from build123d import *

# Parameters (mm, degrees)
SKETCH1_W                                = 152.4
SKETCH1_H                                = 228.6
BOSS_EXTRUDE1_DEPTH                      = 5.588
SKETCH2_R                                = 2.25
SKETCH2_W                                = 22
SKETCH2_H                                = 42
CUT_EXTRUDE1_DEPTH                       = 138.48511099
SKETCH6_R                                = 2.65
CUT_EXTRUDE2_DEPTH                       = 430.910746044
CUT_EXTRUDE3_DEPTH                       = 138.48511099
MIRROR1_AT_THE_SECOND_PLANE_COPY_1_DEPTH = 138.48511099
SKETCH8_R                                = 2.65
CUT_EXTRUDE4_DEPTH                       = 430.910746044
CUT_EXTRUDE5_DEPTH                       = 138.48511099
MIRROR2_AT_THE_SECOND_PLANE_COPY_1_DEPTH = 138.48511099
SKETCH10_W                               = 228.6
SKETCH10_H                               = 5.588
BOSS_EXTRUDE2_DEPTH                      = 25.4
SKETCH11_W                               = 22
SKETCH11_H                               = 42
CUT_EXTRUDE6_DEPTH                       = 154.030309887
CUT_EXTRUDE7_DEPTH                       = 154.030309887
MIRROR5_AT_THE_SECOND_PLANE_COPY_1_DEPTH = 154.030309887


with BuildPart() as part:
    # Sketch1 → Boss-Extrude1 (new body)
    with BuildSketch(Plane(origin=(0, 0, 0), x_dir=(1, 0, 0), z_dir=(0, 1, 0))):
        Rectangle(SKETCH1_W, SKETCH1_H)
    extrude(amount=BOSS_EXTRUDE1_DEPTH)

    # Sketch2 → Cut-Extrude1 (cut, through all)
    with BuildSketch(Plane(origin=(0, 5.588, 0), x_dir=(1, 0, 0), z_dir=(0, 1, 0))):
        with Locations(Location((64.145199836, -6.727348554, 0), (0, 0, 270))):
            Circle(SKETCH2_R)
        with Locations((74.145199836, -6.727348554)):
            Circle(SKETCH2_R)
        with Locations(Location((64.145199836, -54.727348554, 0), (0, 0, 270))):
            Circle(SKETCH2_R)
        with Locations((74.145199836, -54.727348554)):
            Circle(SKETCH2_R)
        with Locations((-74.023936008, -54.727348554)):
            Circle(SKETCH2_R)
        with Locations(Location((-64.023936008, -54.727348554, 0), (0, 0, 90))):
            Circle(SKETCH2_R)
        with Locations((-74.023936008, -6.727348554)):
            Circle(SKETCH2_R)
        with Locations(Location((-64.023936008, -6.727348554, 0), (0, 0, 90))):
            Circle(SKETCH2_R)
        with Locations((69.145199836, -30.727348554)):
            Rectangle(SKETCH2_W, SKETCH2_H)
        with Locations((-69.023936008, -30.727348554)):
            Rectangle(SKETCH2_W, SKETCH2_H)
    extrude(amount=-CUT_EXTRUDE1_DEPTH, mode=Mode.SUBTRACT)

    # Sketch6 → Cut-Extrude2 (cut, through all)
    with BuildSketch(Plane(origin=(-338.200209725, 5.588, 0), x_dir=(1, 0, 0), z_dir=(0, 1, 0))):
        with Locations(Location((404.400209725, 104.3, 0), (0, 0, 270))):
            Circle(SKETCH6_R)
    extrude(amount=-CUT_EXTRUDE2_DEPTH, mode=Mode.SUBTRACT)

    # Sketch7 → Cut-Extrude3 (cut, through all)
    with BuildSketch(Plane(origin=(0, 5.588, 0), x_dir=(1, 0, 0), z_dir=(0, 1, 0))):
        with BuildLine():
            Line((68.85, 105.377738503), (68.85, 97.377738503))
            ThreePointArc((68.85, 97.377738503), (66.2, 94.727738503), (63.55, 97.377738503))
            Line((63.55, 97.377738503), (63.55, 105.377738503))
            ThreePointArc((63.55, 105.377738503), (66.2, 108.027738503), (68.85, 105.377738503))
        make_face()
    cut_extrude3 = extrude(amount=-CUT_EXTRUDE3_DEPTH, mode=Mode.SUBTRACT)

    # Mirror1: Cut-Extrude3 across plane
    add(cut_extrude3.mirror(Plane.XY), mode=Mode.SUBTRACT)

    # Mirror1 at the second plane: Cut-Extrude3 across plane
    add(cut_extrude3.mirror(Plane(origin=(0, 0, 0), x_dir=(0, 0, 1), z_dir=(1, 0, 0))), mode=Mode.SUBTRACT)

    # Mirror1 at the second plane copy 1 sketc → Mirror1 at the second plane copy 1 (cut, through all)
    with BuildSketch(Plane(origin=(0, 5.588, 0), x_dir=(-1, 0, 0), z_dir=(0, 1, 0))):
        with BuildLine():
            Line((68.85, 105.377738503), (68.85, 97.377738503))
            ThreePointArc((68.85, 97.377738503), (66.2, 94.727738503), (63.55, 97.377738503))
            Line((63.55, 97.377738503), (63.55, 105.377738503))
            ThreePointArc((63.55, 105.377738503), (66.2, 108.027738503), (68.85, 105.377738503))
        make_face()
    extrude(amount=-MIRROR1_AT_THE_SECOND_PLANE_COPY_1_DEPTH, mode=Mode.SUBTRACT)

    # Sketch8 → Cut-Extrude4 (cut, through all)
    with BuildSketch(Plane(origin=(-338.200209725, 5.588, 0), x_dir=(1, 0, 0), z_dir=(0, 1, 0))):
        with Locations(Location((381.82832329, 70.726177663, 0), (0, 0, 270))):
            Circle(SKETCH8_R)
    extrude(amount=-CUT_EXTRUDE4_DEPTH, mode=Mode.SUBTRACT)

    # Sketch9 → Cut-Extrude5 (cut, through all)
    with BuildSketch(Plane(origin=(0, 5.588, 0), x_dir=(1, 0, 0), z_dir=(0, 1, 0))):
        with BuildLine():
            Line((43.628113565, 68.076177663), (23.628113565, 68.076177663))
            ThreePointArc((23.628113565, 68.076177663), (20.978113565, 70.726177663), (23.628113565, 73.376177663))
            Line((23.628113565, 73.376177663), (43.628113565, 73.376177663))
            ThreePointArc((43.628113565, 73.376177663), (46.278113565, 70.726177663), (43.628113565, 68.076177663))
        make_face()
    cut_extrude5 = extrude(amount=-CUT_EXTRUDE5_DEPTH, mode=Mode.SUBTRACT)

    # Mirror2: Cut-Extrude5 across plane
    add(cut_extrude5.mirror(Plane.XY), mode=Mode.SUBTRACT)

    # Mirror2 at the second plane: Cut-Extrude5 across plane
    add(cut_extrude5.mirror(Plane(origin=(0, 0, 0), x_dir=(0, 0, 1), z_dir=(1, 0, 0))), mode=Mode.SUBTRACT)

    # Mirror2 at the second plane copy 1 sketc → Mirror2 at the second plane copy 1 (cut, through all)
    with BuildSketch(Plane(origin=(0, 5.588, 0), x_dir=(-1, 0, 0), z_dir=(0, 1, 0))):
        with BuildLine():
            Line((43.628113565, 68.076177663), (23.628113565, 68.076177663))
            ThreePointArc((23.628113565, 68.076177663), (20.978113565, 70.726177663), (23.628113565, 73.376177663))
            Line((23.628113565, 73.376177663), (43.628113565, 73.376177663))
            ThreePointArc((43.628113565, 73.376177663), (46.278113565, 70.726177663), (43.628113565, 68.076177663))
        make_face()
    extrude(amount=-MIRROR2_AT_THE_SECOND_PLANE_COPY_1_DEPTH, mode=Mode.SUBTRACT)

    # Sketch10 → Boss-Extrude2 (add)
    with BuildSketch(Plane.ZY.offset(76.2)):
        with Locations((0, 2.794)):
            Rectangle(SKETCH10_W, SKETCH10_H)
    boss_extrude2 = extrude(amount=BOSS_EXTRUDE2_DEPTH)

    # Sketch11 → Cut-Extrude6 (cut, through all)
    with BuildSketch(Plane(origin=(0, 5.588, 0), x_dir=(1, 0, 0), z_dir=(0, 1, 0))):
        with Locations((-69.023936008, -30.727348554)):
            Rectangle(SKETCH11_W, SKETCH11_H)
    cut_extrude6 = extrude(amount=-CUT_EXTRUDE6_DEPTH, mode=Mode.SUBTRACT)

    # Mirror4: Boss-Extrude2, Cut-Extrude6 across plane
    add(boss_extrude2.mirror(Plane(origin=(0, 0, 0), x_dir=(0, 0, 1), z_dir=(1, 0, 0))))
    add(cut_extrude6.mirror(Plane(origin=(0, 0, 0), x_dir=(0, 0, 1), z_dir=(1, 0, 0))), mode=Mode.SUBTRACT)

    # Sketch12 → Cut-Extrude7 (cut, through all)
    with BuildSketch(Plane(origin=(0, 5.588, 0), x_dir=(1, 0, 0), z_dir=(0, 1, 0))):
        with BuildLine():
            Line((-83.55, -97.377738503), (-83.55, -105.377738503))
            ThreePointArc((-83.55, -105.377738503), (-86.2, -108.027738503), (-88.85, -105.377738503))
            Line((-88.85, -105.377738503), (-88.85, -97.377738503))
            ThreePointArc((-88.85, -97.377738503), (-86.2, -94.727738503), (-83.55, -97.377738503))
        make_face()
    cut_extrude7 = extrude(amount=-CUT_EXTRUDE7_DEPTH, mode=Mode.SUBTRACT)

    # Mirror5: Cut-Extrude7 across plane
    add(cut_extrude7.mirror(Plane(origin=(0, 0, 0), x_dir=(0, 0, 1), z_dir=(1, 0, 0))), mode=Mode.SUBTRACT)

    # Mirror5 at the second plane: Cut-Extrude7 across plane
    add(cut_extrude7.mirror(Plane.XY), mode=Mode.SUBTRACT)

    # Mirror5 at the second plane copy 1 sketc → Mirror5 at the second plane copy 1 (cut, through all)
    with BuildSketch(Plane(origin=(0, 5.588, 0), x_dir=(-1, 0, 0), z_dir=(0, 1, 0))):
        with BuildLine():
            Line((-83.55, -97.377738503), (-83.55, -105.377738503))
            ThreePointArc((-83.55, -105.377738503), (-86.2, -108.027738503), (-88.85, -105.377738503))
            Line((-88.85, -105.377738503), (-88.85, -97.377738503))
            ThreePointArc((-88.85, -97.377738503), (-86.2, -94.727738503), (-83.55, -97.377738503))
        make_face()
    extrude(amount=-MIRROR5_AT_THE_SECOND_PLANE_COPY_1_DEPTH, mode=Mode.SUBTRACT)


solid = part.part
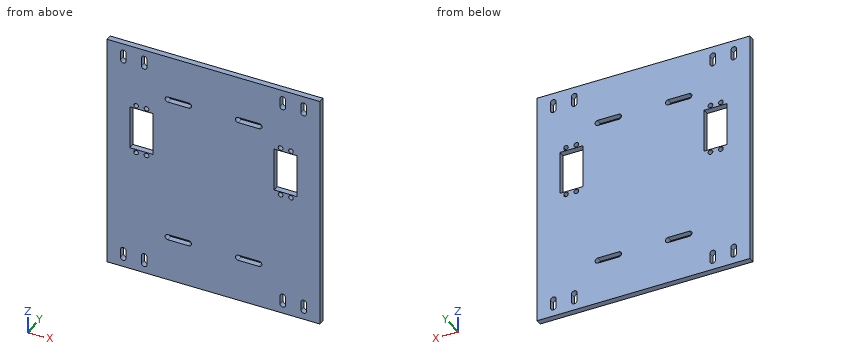
The model under review builds one solid part; all positions refer to its coordinate system, in mm. Coordinates: 2 decimals unless noted, no trailing zeros. Loops run counter-clockwise (first coordinate to the right, second up) from the corner with the lowest first, then second, coordinate; pieces in that order, holes last. Notation, with made-up numbers: M -3,-28 L 16,-28 A17 ccw 16,-11 Z; hole C 12,82.25 d8. An arc over 180 degrees is marked long. Put each result on its own line as item: value. Start each with the question number.
Q1. Add section C-C (y = 2.85). Count the separate pieces of the cut face and the enclosed holes in it, and give its area (3 significant figures).
Q2. Clearance check with a flat-ended pin moving along its axis: pin 1 (4 mm diameter, centred on x = -74.02, z = 6.73, fed in from -Y). State where the tip first meets the part, or that it passes through.
Q3. Wall thickness on line 1 (Z direction, x = 33.5, y = 4.45); line 2 (X direction, y = 3.1, z = 104); line 3 (X direction, y = 3.45, z = 44): over which ranges is each line inside the solid? List them lowest first.
Q4. Add section B-B (z = 37.5). Write out the cut boundary in (x, y).
Q5. Add section A-A (x = 31.5). Write out the cut boundary in (y, z), and give its area (3 significant figures).
Answers:
1. separate pieces: 1
1. enclosed holes: 22
1. area: 43,400 mm^2
2. pin 1: passes through
3. line 1: z = -114.3 to -73.38, -68.08 to 68.08, 73.38 to 114.3
3. line 2: x = -101.6 to -88.85, -83.55 to -68.85, -63.55 to 63.55, 68.85 to 83.55, 88.85 to 101.6
3. line 3: x = -101.6 to -80.02, -58.02 to 58.02, 80.02 to 101.6
4. outline: M -101.6,0 L -80.02,0 L -80.02,5.59 L -101.6,5.59 Z; M -58.02,0 L 58.02,0 L 58.02,5.59 L -58.02,5.59 Z; M 80.02,0 L 101.6,0 L 101.6,5.59 L 80.02,5.59 Z
5. outline: M 0,-114.3 L 5.59,-114.3 L 5.59,-73.38 L 0,-73.38 Z; M 0,-68.08 L 5.59,-68.08 L 5.59,68.08 L 0,68.08 Z; M 0,73.38 L 5.59,73.38 L 5.59,114.3 L 0,114.3 Z
5. area: 1,220 mm^2
